Source: CAD feature listing. Evaluate the final solid. Frame: model axes, mm. Face numbers are marked on the shaded views. Give positions to 0.01 mm unless a question says otherwise; leave off trailing zeros. Order: outer loops, then holes, each group sorted by start corner. A loop starts at its lowest first (then second) coordinate and runs counter-clockwise, first axis right, second up. Notation, with made-up numbers: M -10.5,75 L 24.5,75 A23 ccw 24.5,104 Z; hole C 77,38.5 d11. An arc over 180 degrees is marked long. Answer as a JSON object with one key per item and string values. Group by question number.
1. Section query A-A (x = 0). Output: boundary loops of the cut face in (y, z).
2. Material intervals for L1, parallel to Y at x = 50, z = 2.5; L2, parallel to X at y = -0.5, z = 0.6; L3, parallel to X at y = 0.25, z = 0.9, sorted ascending. Write a range as [from, to].
3. Section query C-C (x = 37.5). Output: boundary loops of the cut face in (y, z), plus the area to 3 significant figures.
4. Pin query (flat end, axial travel): P1, Ø4, axis at x = 0, y = 0, coming from the -Z side; P2, Ø2, axis at y = -3, z = 2.5, coming from the +X side; P3, Ø5, axis at x = 37.5, y = 0, coming from the -Z side. Return the tip coordinate at first contact, or that it passes through.
5. Pull-direction query (Y, two-part tool) for the marked faces 1, 2 and 3; classes: +Y half, -Y half, draft (parallel to the pull), parting line (faces both ways), or undercut.
6. Section query B-B (z = 1.75). Count the separate pieces of the cut face and the enclosed holes in it, plus the area to 3 significant figures.
Autodesk Inventor part; units mm, degrees
ref_plane "YZ Plane" through (0, 0, 0) normal (1, 0, 0) x (0, 1, 0)
ref_plane "XZ Plane" through (0, 0, 0) normal (0, 1, 0) x (-1, 0, 0)
ref_plane "XY Plane" through (0, 0, 0) normal (0, 0, 1) x (1, 0, 0)
sketch "Sketch1" plane through (0, 0, 0) normal (0, 0, 1) x (1, 0, 0)
  circle A0 centre (0, 0) radius 3.15
  line L0 (0, 0) -> (50, 0) construction
  line L1 (0, -9) -> (50, -9)
  line L2 (50, 9) -> (0, 9)
  arc A1 (0, 9) -> (0, -9) centre (0, 0) ccw
  arc A2 (50, -9) -> (50, 9) centre (50, 0) ccw
  line L3 (0, 0) -> (50, 0) construction
  circle A3 centre (50, 0) radius 1.5
  circle A4 centre (37.5, 0) radius 1.5
  circle A5 centre (-5.7956, -1.5529) radius 1.5
  circle A6 centre (-5.7956, 1.5529) radius 1.5
  line L4 (0, 0) -> (-5.7956, 1.5529) construction
  line L5 (0, 0) -> (-5.7956, -1.5529) construction
  line L6 (0, 0) -> (-9, 0) construction
  arc A7 (-4.3467, 1.1647) -> (-4.3467, -1.1647) centre (0, 0) ccw
  arc A8 (-7.2444, 1.9411) -> (-7.2444, -1.9411) centre (0, 0) ccw
  line L7 (-1.8674, 2.5368) -> (1.2741, 2.8808)
  point P0 (25, 0)
  dimension "d0" = 6.3
  dimension "d1" = 50
  dimension "d2" = 0
  dimension "d3" = 18
  dimension "d4" = 3
  dimension "d5" = 3
  dimension "d6" = 12.5
  dimension "d7" = 3
  dimension "d8" = 3
  dimension "d9" = 15
  dimension "d10" = 15
  dimension "d12" = 6
  dimension "d15" = 2.725
  dimension "d16" = -6.25
  dimension "d17" = 6
extrude "Extrusion1" add sketch "Sketch1" along normal blind 6
sketch "Sketch2" plane through (0, 0, 0) normal (0, 0, -1) x (-1, 0, 0)
  arc A0 (-50, 9) -> (-50, -9) centre (-50, 0) ccw
  line L0 (0, -9) -> (-50, -9)
  arc A1 (0, -9) -> (0, 9) centre (0, 0) ccw
  line L1 (-50, 9) -> (0, 9)
  circle A2 centre (-37.5, 0) radius 1.5
  arc A3 (7.2444, -1.9411) -> (7.2444, 1.9411) centre (0, 0) ccw
  arc A4 (4.3467, -1.1647) -> (7.2444, -1.9411) centre (5.7956, -1.5529) ccw
  arc A5 (4.3467, -1.1647) -> (4.3467, 1.1647) centre (0, 0) ccw
  arc A6 (7.2444, 1.9411) -> (4.3467, 1.1647) centre (5.7956, 1.5529) ccw
  circle A7 centre (-50, 0) radius 1.5
  circle A8 centre (0, 0) radius 3.15
  line L2 (9, 5) -> (-59, 5)
  line L3 (-59, 5) -> (-59, -5)
  line L4 (-59, -5) -> (9, -5)
  line L5 (9, -5) -> (9, 5)
  circle A9 centre (-50, 0) radius 5
  point P0 (7.4833, -5)
  point P1 (-50, -5)
  point P2 (-50, 5)
  point P3 (7.4833, 5)
  dimension "d18" = 5
  dimension "d19" = 10
  dimension "d20" = 9
  dimension "d21" = 59
extrude "Extrusion2" cut sketch "Sketch2" against normal blind 6 contours L1 A1 L2 A0 | L2 A9 L4 A0 | L4 A1 L0 A0
fillet "Fillet1" radius 5 2 edges at (-7.4833, 5, 3) (-7.4833, -5, 3)
sketch "Sketch3" plane through (0, 0, 6) normal (0, 0, 1) x (1, 0, 0)
  circle A0 centre (0, 0) radius 3.15
  circle A1 centre (50, 0) radius 1.5
  arc A2 (-7.2444, 1.9411) -> (-7.2444, -1.9411) centre (0, 0) ccw
  arc A3 (-4.3467, 1.1647) -> (-7.2444, 1.9411) centre (-5.7956, 1.5529) ccw
  arc A4 (-4.3467, 1.1647) -> (-4.3467, -1.1647) centre (0, 0) ccw
  arc A5 (-7.2444, -1.9411) -> (-4.3467, -1.1647) centre (-5.7956, -1.5529) ccw
  circle A6 centre (37.5, 0) radius 1.5
properties part number "Arm2_3D" material "Aluminum 6061, Welded"
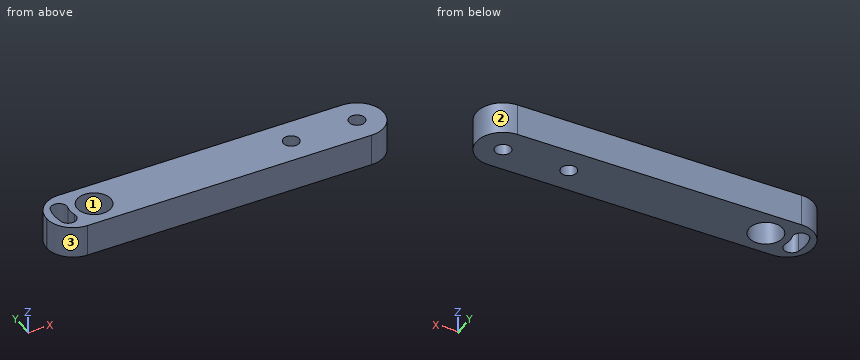
Answer sheet:
{
 "1": {"outline": "M -5,0 L -3.15,0 L -3.15,6 L -5,6 Z; M 3.15,0 L 5,0 L 5,6 L 3.15,6 Z"},
 "2": {"L1": "[-5, -1.5], [1.5, 5]", "L2": "[-8.97, -7.48], [-4.47, -3.11], [3.11, 36.09], [38.91, 48.59], [51.41, 54.97]", "L3": "[-8.99, -7.5], [-4.49, -3.14], [3.14, 36.02], [38.98, 48.52], [51.48, 54.99]"},
 "3": {"outline": "M -5,0 L -1.5,0 L -1.5,6 L -5,6 Z; M 1.5,0 L 5,0 L 5,6 L 1.5,6 Z", "area": "42.0 mm^2"},
 "4": {"P1": "through", "P2": "x = 54.58", "P3": "z = 0"},
 "5": {"face 1": "undercut", "face 2": "parting line", "face 3": "-Y half"},
 "6": {"separate pieces": "1", "enclosed holes": "4", "area": "557 mm^2"}
}
